The listing builds one solid part. Answer for the finished solid, in the listing's coordinates (mm). Coordinates: 2 decimals unless noted, no trailing zeros. Write each loop counter-clockwise with the first axis right and the second up, starting at its lowest first coordinate (ties: lowest second). Pieces come first, ordered by that corner, then holes.
from build123d import *

# Parameters (mm, degrees)
SKETCH1_W                                           = 240
SKETCH1_H                                           = 180
EXTRUDE1_DEPTH                                      = 20
CBORE_FOR_M6_HEX_SOCKET_HEAD_CAP_SCREW1_D           = 6.6
CBORE_FOR_M6_HEX_SOCKET_HEAD_CAP_SCREW1_CBORE_D     = 11
CBORE_FOR_M6_HEX_SOCKET_HEAD_CAP_SCREW1_CBORE_DEPTH = 6.4


with BuildPart() as part:
    # Sketch1 → Extrude1 (new body)
    with BuildSketch(Plane.XY):
        Rectangle(SKETCH1_W, SKETCH1_H)
    extrude(amount=EXTRUDE1_DEPTH)

    # CBORE for M6 Hex Socket Head Cap Screw1 (through all)
    with Locations(Plane(origin=(0, 0, 0), x_dir=(-1, 0, 0), z_dir=(0, 0, -1))):
        with Locations((-90, 75), (-90, -75), (-90, -15), (90, -15), (90, -75), (90, 75)):
            CounterBoreHole(CBORE_FOR_M6_HEX_SOCKET_HEAD_CAP_SCREW1_D / 2, CBORE_FOR_M6_HEX_SOCKET_HEAD_CAP_SCREW1_CBORE_D / 2, CBORE_FOR_M6_HEX_SOCKET_HEAD_CAP_SCREW1_CBORE_DEPTH)


solid = part.part
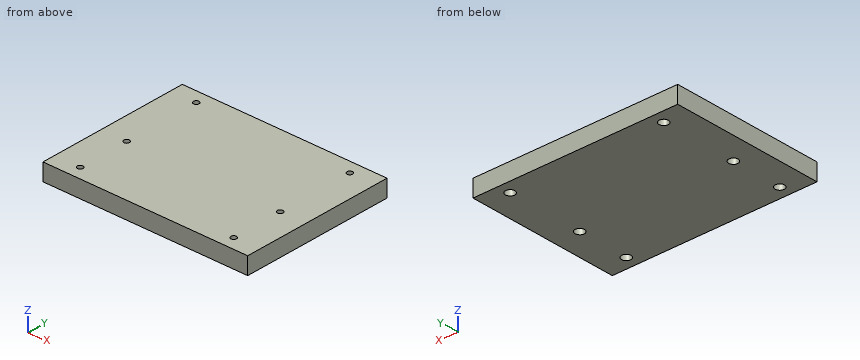
1. Find the intervals of material crossed by L1, parallel to Y at x = -90, z = 3.75; L2, parallel to Y at x = -90, z = 9.75, in increasing order.
Results found:
L1: y = -90 to -80.5, -69.5 to -20.5, -9.5 to 69.5, 80.5 to 90
L2: y = -90 to -78.3, -71.7 to -18.3, -11.7 to 71.7, 78.3 to 90
2. Section A-A on x = -90 is taken. Give the vertices of the cut face in (y, z).
Results found:
outline: (-90, 0) - (-80.5, 0) - (-80.5, 6.4) - (-78.3, 6.4) - (-78.3, 20) - (-90, 20) - close; (-71.7, 6.4) - (-69.5, 6.4) - (-69.5, 0) - (-20.5, 0) - (-20.5, 6.4) - (-18.3, 6.4) - (-18.3, 20) - (-71.7, 20) - close; (-11.7, 6.4) - (-9.5, 6.4) - (-9.5, 0) - (69.5, 0) - (69.5, 6.4) - (71.7, 6.4) - (71.7, 20) - (-11.7, 20) - close; (78.3, 6.4) - (80.5, 6.4) - (80.5, 0) - (90, 0) - (90, 20) - (78.3, 20) - close
3. Section B-B on y = -15 is taken. Give the vertices of the cut face in (x, z), then the cut area to 3 significant figures.
Results found:
outline: (-120, 0) - (-95.5, 0) - (-95.5, 6.4) - (-93.3, 6.4) - (-93.3, 20) - (-120, 20) - close; (-86.7, 6.4) - (-84.5, 6.4) - (-84.5, 0) - (84.5, 0) - (84.5, 6.4) - (86.7, 6.4) - (86.7, 20) - (-86.7, 20) - close; (93.3, 6.4) - (95.5, 6.4) - (95.5, 0) - (120, 0) - (120, 20) - (93.3, 20) - close
area: 4,480 mm2
4. A flat-ended cylindrical pin translates along its axis: P1, Ø3.5, axis at x = 90.5, y = -16.5, coming from the -Z side. Find the tip coordinate at first contact, or state that the pin passes through.
Results found:
P1: stops at z = 6.4
